from build123d import *

# Parameters (mm, degrees)
SKETCH1_W           = 24
SKETCH1_H           = 20
BOSS_EXTRUDE1_DEPTH = 3
SKETCH3_R           = 1.6
CUT_EXTRUDE1_DEPTH  = 4
CUT_EXTRUDE2_DEPTH  = 1.5
FILLET1_R           = 10


with BuildPart() as part:
    # Sketch1 → Boss-Extrude1 (new body)
    with BuildSketch(Plane.XY):
        with Locations((0, 10)):
            Rectangle(SKETCH1_W, SKETCH1_H)
    extrude(amount=BOSS_EXTRUDE1_DEPTH)

    # Sketch3 → Cut-Extrude1 (cut, through all)
    with BuildSketch(Plane.XY.offset(3)):
        with Locations((0, 5)):
            Circle(SKETCH3_R)
    extrude(amount=-CUT_EXTRUDE1_DEPTH, mode=Mode.SUBTRACT)

    # Sketch2 → Cut-Extrude2 (cut)
    with BuildSketch(Plane.XY.offset(3)):
        with BuildLine():
            Line((-12, 14.851322054), (-12, 20))
            Line((-12, 20), (12, 20))
            Line((12, 20), (12, 14.851322054))
            ThreePointArc((12, 14.851322054), (0, 14), (-12, 14.851322054))
        make_face()
    extrude(amount=-CUT_EXTRUDE2_DEPTH, mode=Mode.SUBTRACT)

    # Fillet1
    fillet1_edges = [part.edges().sort_by_distance(p)[0] for p in [
        (12, 0, 1.5),
        (-12, 0, 1.5),
    ]]
    fillet(fillet1_edges, radius=FILLET1_R)


solid = part.part
Work out the finished part from the listing and answer in its coordinate system (mm). A direction names the side the tool comes from. Give positions to 0.01 mm unless a question says otherwise; leave off trailing zeros. Order: outer loops, then holes, each group sorted by start corner. A loop starts at its lowest first (then second) coordinate and runs counter-clockwise, first axis right, second up. Notation, with made-up numbers: M 81.5,35.5 L 100.5,35.5 A6 ccw 100.5,45.5 Z; hole C 52,-20 d6. An arc over 180 degrees is marked long. Return JSON: item names as keys, results as strings.
Q1. Which of the six approach directions +Z, -Z, +X, -X, +Y, -Y give full straight-line access (tool end or side, diameter ignored) to faces 1 (the face through (0, 14, 2)), 2 (the face through (0, 8, 3))?
Answer below:
{"face 1": "+Z, +Y", "face 2": "+Z, +X, -X, +Y, -Y"}
Q2. Find section A-A, the plane x = 0. Write down the section's boundary in (y, z).
Answer below:
{"outline": "M 0,0 L 3.4,0 L 3.4,3 L 0,3 Z; M 6.6,0 L 20,0 L 20,1.5 L 14,1.5 L 14,3 L 6.6,3 Z"}
Q3. Find section C-C, the plane y = 5. Write down the section's boundary in (x, z), and give its area (3 significant figures).
Answer below:
{"outline": "M -10.66,0 L -1.6,0 L -1.6,3 L -10.66,3 Z; M 1.6,0 L 10.66,0 L 10.66,3 L 1.6,3 Z", "area": "54.4 mm^2"}
Q4. Find section D-D, the plane z = 0.7. Write down the section's boundary in (x, y).
Answer below:
{"outline": "M -12,10 A10 ccw -2,0 L 2,0 A10 ccw 12,10 L 12,20 L -12,20 Z; hole C 0,5 d3.2"}
Q5. The mould has two halves that part along X. Classify faces 3 (the face through (0, 0, 1)), 4 (the face through (-0.35, 3.44, 1.52)), 5 (the face through (12, 14, 1)), 6 (the face through (-9.15, 3.01, 1.52)): pulls with the +X half, pulls with the -X half, needs draft (parallel to the pull), parting line crosses it, or undercut.
Answer below:
{"face 3": "needs draft", "face 4": "undercut", "face 5": "pulls with the +X half", "face 6": "pulls with the -X half"}
Q6. Find section B-B, the plane z = 2.6. Write down the section's boundary in (x, y), and give its area (3 significant figures).
Answer below:
{"outline": "M -12,10 A10 ccw -2,0 L 2,0 A10 ccw 12,10 L 12,14.85 A85 cw -12,14.85 Z; hole C 0,5 d3.2", "area": "292 mm^2"}
Q7. Find the intervals of material crossed by line 1 along Y through (x, z) = (0, 1.9); line 2 along Y through (x, z) = (0, 1.2); line 3 along Z through (x, y) = (-2.5, 14.5), in increasing order. Write a range as [from, to].
Answer below:
{"line 1": "y = [0, 3.4], [6.6, 14]", "line 2": "y = [0, 3.4], [6.6, 20]", "line 3": "z = [0, 1.5]"}
